from build123d import *

# Parameters (mm, degrees)
BOSS_EXTRUDE1_DEPTH = 19.05
FILLET2_R           = 2.54


with BuildPart() as part:
    # Sketch1 → Boss-Extrude1 (new body)
    with BuildSketch(Plane.XY):
        with BuildLine():
            ThreePointArc((101.6, 10.9855), (96.7105, 15.875), (101.6, 20.7645))
            Line((101.6, 20.7645), (101.6, 31.75))
            Line((101.6, 31.75), (38.1, 31.75))
            Line((38.1, 31.75), (38.1, 17.875))
            ThreePointArc((38.1, 17.875), (39.514213562, 17.289213562), (40.1, 15.875))
            ThreePointArc((40.1, 15.875), (39.514213562, 14.460786438), (38.1, 13.875))
            Line((38.1, 13.875), (38.1, 0))
            Line((38.1, 0), (101.6, 0))
            Line((101.6, 0), (101.6, 10.9855))
        make_face()
        with BuildLine():
            Line((101.6, 31.75), (101.6, 20.7645))
            ThreePointArc((101.6, 20.7645), (105.057398607, 19.332398607), (106.4895, 15.875))
            ThreePointArc((106.4895, 15.875), (105.057398607, 12.417601393), (101.6, 10.9855))
            Line((101.6, 10.9855), (101.6, 0))
            Line((101.6, 0), (152.4, 0))
            Line((152.4, 0), (152.4, 25.4))
            Line((152.4, 25.4), (142.875, 25.4))
            Line((142.875, 25.4), (142.875, 12.7))
            Line((142.875, 12.7), (133.35, 12.7))
            Line((133.35, 12.7), (133.35, 31.75))
            Line((133.35, 31.75), (101.6, 31.75))
        make_face()
        with BuildLine():
            Line((38.1, 17.875), (38.1, 31.75))
            Line((38.1, 31.75), (0, 31.75))
            Line((0, 31.75), (0, 0))
            Line((0, 0), (38.1, 0))
            Line((38.1, 0), (38.1, 13.875))
            ThreePointArc((38.1, 13.875), (36.1, 15.875), (38.1, 17.875))
        make_face()
    extrude(amount=BOSS_EXTRUDE1_DEPTH)

    # Fillet2
    fillet2_edges = [part.edges().sort_by_distance(p)[0] for p in [
        (76.2, 0, 19.05),
        (66.675, 31.75, 0),
        (133.35, 22.225, 0),
        (138.1125, 12.7, 0),
        (142.875, 19.05, 0),
        (147.6375, 25.4, 0),
        (152.4, 12.7, 0),
        (152.4, 12.7, 19.05),
        (76.2, 0, 0),
        (0, 15.875, 0),
        (147.6375, 25.4, 19.05),
        (0, 31.75, 9.525),
        (133.35, 31.75, 9.525),
        (133.35, 12.7, 9.525),
        (142.875, 12.7, 9.525),
        (142.875, 25.4, 9.525),
        (152.4, 25.4, 9.525),
        (152.4, 0, 9.525),
        (0, 0, 9.525),
        (142.875, 19.05, 19.05),
        (138.1125, 12.7, 19.05),
        (133.35, 22.225, 19.05),
        (66.675, 31.75, 19.05),
        (0, 15.875, 19.05),
    ]]
    fillet(fillet2_edges, radius=FILLET2_R)


solid = part.part
Model file for the job. Use its own axes, mm. A direction names the side the tool comes from. Round coordinates to 2 decimals unless told otherwise and drop trailing zeros.
(1) Band-saw the part on A-A (z = 12.5). Give the number of separate pieces and of enclosed holes in the cut face, then the cut area to 3 significant figures.
(2) Drill centre lines: line 1 (X direction, y = 18.5, z = 4.75) (3 decimals); line 2 (X direction, y = 21, z = 12) (3 decimals); line 3 (X direction, y = 26.5, z = 7.25). Where is each one in solid material? Low to high.
(3) Pull direction X, two halves, no side cores. Call faces 6 (the face through (0.724, 0.764, 9.623)), 7 (the face through (143.599, 18.997, 0.764)), 8 (the face through (151.676, 0.764, 9.623)): released by +X, released by -X, zero draft, split by the parting line, or undercut.
(4) Pin check, flat tips, straight feed: pin 1 (3.5 mm diameter, centred on x = 137.5, z = 11, fed in from +Y); pin 2 (1.3 mm diameter, centred on x = 147, z = 10, fed in from +Y). Stop position of each tip, or through.
(5) 3-axis set-ups, long thin cutter, end or side, ignore diameter. For faces 1 (the face through (151.676, 12.842, 0.764)), 2 (the face through (143.599, 18.997, 18.286)), 3 (the face through (147.606, 24.676, 18.286)), 4 (the face through (148, 25.4, 9)), 5 (the face through (138.081, 11.976, 0.764)): which of +Z, -Z, +X, -X, +Y, -Y reach the whole face in a straight line?
Verdict:
1. separate pieces: 1
1. enclosed holes: 2
1. area: 4,500 mm2
2. line 1: x = 0 to 97.475, 105.725 to 133.35, 142.875 to 152.4
2. line 2: x = 0 to 133.35, 142.875 to 152.4
2. line 3: x = 0 to 133.35
3. face 6: released by -X
3. face 7: undercut
3. face 8: released by +X
4. pin 1: stops at y = 12.7
4. pin 2: stops at y = 25.4
5. face 1: -Z, +X, +Y, -Y
5. face 2: +Z, +Y
5. face 3: +Z, +X, +Y
5. face 4: +Z, -Z, +X, +Y
5. face 5: -Z, +Y
